```python
from build123d import *

# Parameters (mm, degrees)
EXTRUDE_15_DEPTH         = 15
CUT_EXTRUDE_1_DEPTH      = 146.773797371
CUT_EXTRUDE_1_DEPTH_BACK = 146.773797371
SKETCH_2_R               = 1.75
SKETCH_2_W               = 31
SKETCH_2_H               = 3


with BuildPart() as part:
    # 草图1 → 15台 (new body)
    with BuildSketch(Plane(origin=(0, 0, 0), x_dir=(1, 0, 0), z_dir=(0, 1, 0))):
        Polygon((40, 105), (100, 45), (100, -45), (40, -105), (-40, -105), (-100, -45), (-100, 45), (-40, 105), align=None)
        Polygon((-80, -36.715728753), (-80, 36.715728753), (-51.715728753, 65), (51.715728753, 65), (80, 36.715728753), (80, -36.715728753), (51.715728753, -65), (-51.715728753, -65), align=None, mode=Mode.SUBTRACT)
    extrude(amount=EXTRUDE_15_DEPTH)

    # 草图2 → 切除-拉伸1 (cut, two sides: drawn at the far end of the back side and taken through both)
    with BuildSketch(Plane(origin=(0, 15, 0), x_dir=(1, 0, 0), z_dir=(0, 1, 0)).offset(-CUT_EXTRUDE_1_DEPTH_BACK)):
        with Locations(Location((-74.289321881, -56.568542495, 0), (0, 0, 270))):
            Circle(SKETCH_2_R)
        with Locations(Location((74.289321881, 56.568542495, 0), (0, 0, 270))):
            Circle(SKETCH_2_R)
        with Locations(Location((-74.289321881, 56.568542495, 0), (0, 0, 270))):
            Circle(SKETCH_2_R)
        with Locations(Location((74.289321881, -56.568542495, 0), (0, 0, 270))):
            Circle(SKETCH_2_R)
        with Locations((0, 103.5)):
            Rectangle(SKETCH_2_W, SKETCH_2_H)
        with Locations((0, 66.5)):
            Rectangle(SKETCH_2_W, SKETCH_2_H)
        with Locations((0, -66.5)):
            Rectangle(SKETCH_2_W, SKETCH_2_H)
        with Locations((0, -103.5)):
            Rectangle(SKETCH_2_W, SKETCH_2_H)
    extrude(amount=CUT_EXTRUDE_1_DEPTH + CUT_EXTRUDE_1_DEPTH_BACK, mode=Mode.SUBTRACT)


solid = part.part
```
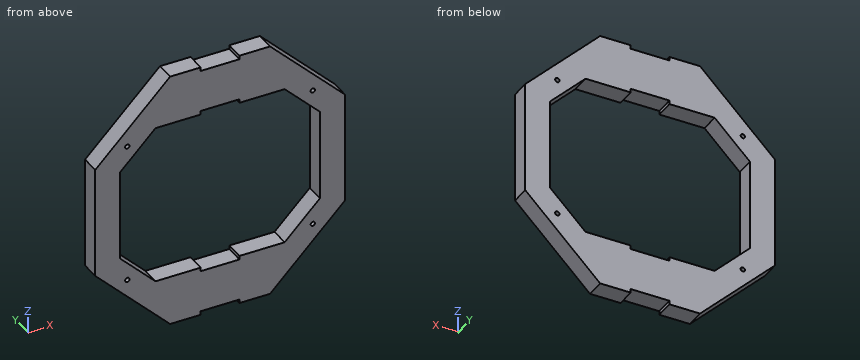
The listing builds one solid part. Answer for the finished solid, in the listing's coordinates (mm). Round coordinates to 2 decimals unless told otherwise and drop trailing zeros. Write each loop counter-clockwise with the first axis right and the second up, starting at its lowest first coordinate (ties: lowest second). Pieces come first, ordered by that corner, then holes. Notation, with made-up numbers: (36.25, 46) -> (54.25, 46) arc R28 ccw to (54.25, 70) -> close; hole circle Ø6 at (82, -9). An arc over 180 degrees is marked (long way). Write item = value, one per line.
1) Given pin 1 (7.5 mm diameter, centred on x = 7, y = 9.5, fed in from +Z); pin 2 (2.5 mm diameter, centred on y = 8.5, z = -104, fed in from -X); pin 3 (2.5 mm diameter, centred on y = 6.5, z = -103, fed in from +X); pin 4 (8 mm diameter, centred on x = -73, z = 82, fed in from +Y), each flat-ended and moving along its own axis, determine where each tip first touches the part or whether it passes through.
Check values:
pin_1 = 102
pin_2 = -42.25
pin_3 = 43.25
pin_4 = through
2) Section C-C on z = 71.5 is taken. Write down the section's boundary in (x, y).
Check values:
outline = (-73.5, 0) -> (73.5, 0) -> (73.5, 15) -> (-73.5, 15) -> close
3) Section D-D on y = 11 is taken. Give the number of separate pieces and of enclosed holes in the cut face, plus the area to 3 significant figures.
Check values:
separate_pieces = 1
enclosed_holes = 5
area = 15,200 mm²
4) Section A-A on x = -8 is taken. Write down the section's boundary in (y, z), plus the area to 3 significant figures.
Check values:
outline = (0, -102) -> (15, -102) -> (15, -68) -> (0, -68) -> close; (0, 68) -> (15, 68) -> (15, 102) -> (0, 102) -> close
area = 1,020 mm²
5) Section B-B on z = -23.5 is taken. Write down the section's boundary in (x, y), plus the area to 3 significant figures.
Check values:
outline = (-100, 0) -> (-80, 0) -> (-80, 15) -> (-100, 15) -> close; (80, 0) -> (100, 0) -> (100, 15) -> (80, 15) -> close
area = 600 mm²
6) Straight lines are drawn through the part: line 1 along Z through (x, y) = (-25.5, 6.25); line 2 along X through (y, z) = (7.5, 22); line 3 along Z through (x, y) = (10, 7.5). For each, find the intervals that lie inside material, in ascending order. Write a range as [from, to].
Check values:
line_1 = [-105, -65], [65, 105]
line_2 = [-100, -80], [80, 100]
line_3 = [-102, -68], [68, 102]
